Input: dimensioned drawing with shaded views. Units: mm. Origin: part minimum x, y, z. Round coordinates to 2 decimals unless told otherwise and drop trailing zeros. Write item = value, one per line. Start each with the question number.
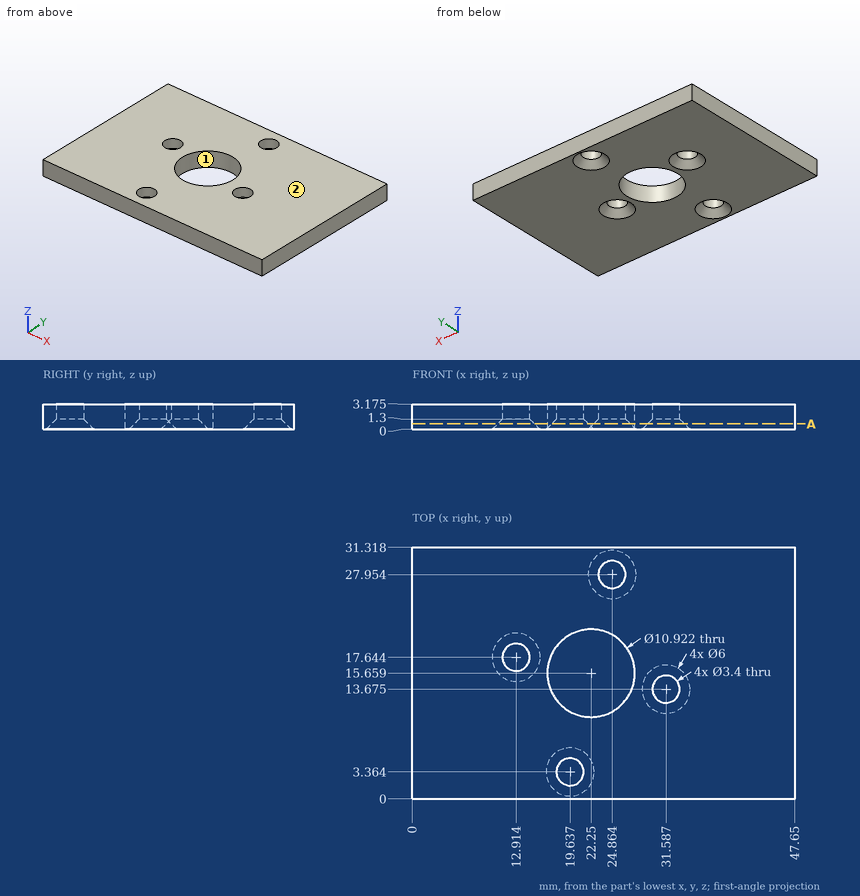
(1) Ray query, L1, parallel to Y at x = 12.5, z = 1.75 (1 decimal); L2, parallel to X at y = 15.5, z = 2.55; L3, parallel to Y at x = 13, z = 0.95 (1 decimal). Return the intervals inside material, ascending. Write a range as from..to.
(2) Contact query for a flat-ended pin moving along its axis: P1, Ø8.5, axis at x = 22.25, y = 15.66, coming from the -Z side. Output: stop coordinate, or through.
(3) Pull-direction query (Y, two-part tool) for the marked faces 1 and 2; classes: +Y half, -Y half, draft (parallel to the pull), parting line (faces both ways), or undercut.
(4) Section A-A (z = 0.7). Count the separate pieces of the cut face and the enclosed holes in it, plus the area to 3 significant figures.
Solution:
q1.L1 = 0..16, 19.3..31.3
q1.L2 = 0..16.79, 27.71..47.65
q1.L3 = 0..15.6, 19.7..31.3
q2.P1 = through
q3.face_1 = undercut
q3.face_2 = draft
q4.separate_pieces = 1
q4.enclosed_holes = 5
q4.area = 1,330 mm^2
